Can you work these out from the model? Positions are in its coordinate system, mm. A direction names the side the tool comes from. Round coordinates to 2 decimals unless told otherwise and drop trailing zeros. Order: outer loops, then holes, each group sorted by start corner. A loop starts at its lowest first (then second) coordinate and runs counter-clockwise, first axis right, second up. Notation, with made-up numbers: M 43.25,5.5 L 50.25,5.5 A16 ccw 50.25,24.5 Z; hole C 84.25,20 d11. An arc over 180 degrees is marked long. One line per question, with ' | ' between items.
```python
from build123d import *

# Parameters (mm, degrees)
BOSS_EXTRUDE1_DEPTH = 2.54
SKETCH2_R           = 2.159
CUT_EXTRUDE1_DEPTH  = 2.54
FILLET1_R           = 5.08
SKETCH3_W           = 2.54
SKETCH3_H           = 6.35
CUT_EXTRUDE4_DEPTH  = 3.54


with BuildPart() as part:
    # Sketch1 → Boss-Extrude1 (new body)
    with BuildSketch(Plane.XY):
        Polygon((67.0433, -78.881), (67.0433, 48.881), (-67.0433, 48.881), (-67.0433, -78.881), (-97.0433, -78.881), (-97.0433, 78.881), (97.0433, 78.881), (97.0433, -78.881), align=None)
    extrude(amount=BOSS_EXTRUDE1_DEPTH)

    # Sketch2 → Cut-Extrude1 (cut)
    with BuildSketch(Plane.XY.offset(2.54)):
        with Locations((-87.6643, 68.2485)):
            Circle(SKETCH2_R)
        with Locations((-87.6643, 58.4695)):
            Circle(SKETCH2_R)
        with Locations((-39.4043, 68.2485)):
            Circle(SKETCH2_R)
        with Locations((-39.4043, 58.4695)):
            Circle(SKETCH2_R)
        Polygon((-42.9603, 73.4555), (-84.1083, 73.4555), (-84.1083, 53.2625), (-42.9603, 53.2625), (-42.9603, 63.359), align=None)
    extrude(amount=-CUT_EXTRUDE1_DEPTH, mode=Mode.SUBTRACT)

    # Fillet1
    fillet1_edges = [part.edges().sort_by_distance(p)[0] for p in [
        (-97.0433, 78.881, 1.27),
        (97.0433, 78.881, 1.27),
        (67.0433, -78.881, 1.27),
        (-67.0433, -78.881, 1.27),
    ]]
    fillet(fillet1_edges, radius=FILLET1_R)

    # Sketch3 → Cut-Extrude4 (cut, through all)
    with BuildSketch(Plane.XY.offset(2.54)):
        with Locations((-84.1083, 63.359)):
            Rectangle(SKETCH3_W, SKETCH3_H)
    extrude(amount=-CUT_EXTRUDE4_DEPTH, mode=Mode.SUBTRACT)


solid = part.part
```
(1) If we section it at D-D on x = 12: Please give me the cut outline in (y, z), plus the area to 3 significant figures.
Final values:
outline: M 48.88,0 L 78.88,0 L 78.88,2.54 L 48.88,2.54 Z | area: 76.2 mm^2
(2) If we section it at A-A on y = -49: Please give me the cut outline in (x, z), plus the area to 3 significant figures.
Final values:
outline: M -97.04,0 L -67.04,0 L -67.04,2.54 L -97.04,2.54 Z; M 67.04,0 L 97.04,0 L 97.04,2.54 L 67.04,2.54 Z | area: 152 mm^2
(3) Thinking about a two-plate mould opening in Y: for faces 3 (the cylindrical face through (-39.69, 60.61, 1.29)), 4 (the flat face through (1, 54, 2.54)), 5 (the cylindrical face through (-68.49, -77.35, 1.29)), 6 (the cylindrical face through (-86.67, 66.33, 1.29)), which applies, released by +Y, released by -Y, zero draft, split by the parting line, or undercut?
Final values:
face 3: undercut | face 4: zero draft | face 5: released by -Y | face 6: undercut
(4) Please list where these lines run through material, in increasing order: probe 1 along Y at (x, z) = (-39, 0.6); probe 2 along X at (y, z) = (-15, 2.45); probe 3 along Y at (x, z) = (-78, 0.5). Write a range as [from, to].
Final values:
probe 1: [48.88, 56.35], [60.59, 66.13], [70.37, 78.88] | probe 2: [-97.04, -67.04], [67.04, 97.04] | probe 3: [-78.88, 53.26], [73.46, 78.88]
(5) On a 3-axis mill with a long thin cutter (end or side, diameter ignored), from which of +Z, -Z, +X, -X, +Y, -Y can I reach the whole of each face in a straight line? I mean faces 1 (the cylindrical face through (68.49, -77.35, 1.29)), 2 (the cylindrical face through (95.595, 77.353, 1.288)). Say none if no direction works.
Final values:
face 1: +Z, -Z, -Y | face 2: +Z, -Z, +X, +Y
(6) If we section it at C-C on z = 0.5: Please give me the cut outline in (x, y).
Final values:
outline: M -97.04,-78.88 L -72.12,-78.88 A5.08 ccw -67.04,-73.8 L -67.04,48.88 L 67.04,48.88 L 67.04,-73.8 A5.08 ccw 72.12,-78.88 L 97.04,-78.88 L 97.04,73.8 A5.08 ccw 91.96,78.88 L -91.96,78.88 A5.08 ccw -97.04,73.8 Z; hole C -87.66,58.47 d4.32; hole C -87.66,68.25 d4.32; hole M -85.38,60.18 L -84.11,60.18 L -84.11,53.26 L -42.96,53.26 L -42.96,73.46 L -84.11,73.46 L -84.11,66.53 L -85.38,66.53 Z; hole C -39.4,58.47 d4.32; hole C -39.4,68.25 d4.32
(7) If we section it at B-B on x = -53.5: Please give me the cut outline in (y, z), plus the area to 3 significant figures.
Final values:
outline: M 48.88,0 L 53.26,0 L 53.26,2.54 L 48.88,2.54 Z; M 73.46,0 L 78.88,0 L 78.88,2.54 L 73.46,2.54 Z | area: 24.9 mm^2
(8) Will this pin go through, and if not, where does the flat tip stop? pin 1 Ø1.3 at (x, z) = (32.5, 0.5) entering from -Y.
Final values:
pin 1: y = 48.88
